Autodesk Inventor part; units mm, degrees
ref_plane "YZ Plane" through (0, 0, 0) normal (1, 0, 0) x (0, 1, 0)
ref_plane "XZ Plane" through (0, 0, 0) normal (0, 1, 0) x (-1, 0, 0)
ref_plane "XY Plane" through (0, 0, 0) normal (0, 0, 1) x (1, 0, 0)
sketch "Sketch1" plane through (0, 0, 0) normal (0, 0, 1) x (1, 0, 0)
  line L0 (0, 0) -> (20, 0)
  line L1 (20, 0) -> (20, -16)
  line L2 (20, -16) -> (0, -16)
  line L3 (0, -16) -> (0, 0)
  circle A0 centre (10, -8) radius 2.5
  dimension "d0" = 20
  dimension "d1" = 16
  dimension "d2" = 8
  dimension "d3" = 10
  dimension "d4" = 5
extrude "Extrusion1" add sketch "Sketch1" along normal blind 5
sketch "Sketch2" plane through (0, 0, 0) normal (0, 1, 0) x (1, 0, 0)
  line L0 (20, 0) -> (20, -5)
  line L1 (20, 0) -> (30, 0)
  line L2 (30, 0) -> (30, 7.76)
  line L3 (30, 7.76) -> (20, 7.76)
  line L4 (20, 7.76) -> (20, 0)
  line L5 (20, -5) -> (30, -5)
  line L6 (30, -5) -> (30, 0)
  line L7 (30, 0) -> (20, 0)
  line L8 (20, 0) -> (20, -5)
  circle A0 centre (25, 3.88) radius 2.6
  point P0 (0, 0)
  dimension "d7" = 10
  dimension "d8" = 7.76
  dimension "d9" = 5.2
extrude "Extrusion2" add sketch "Sketch2" against normal blind 16
sketch "Sketch3" plane through (0, -16, 0) normal (0, -1, 0) x (1, 0, 0)
  line L0 (30, -7.76) -> (30, 5)
  line L1 (0, 0) -> (20, 0)
  line L2 (30, -7.76) -> (20, -7.76)
  line L3 (20, -7.76) -> (20, 0)
  line L4 (20, 0) -> (30, 0)
  line L5 (30, 0) -> (30, -7.76)
extrude "Extrusion3" add sketch "Sketch3" against normal blind 9
sketch "Sketch4" plane through (0, -16, 0) normal (0, -1, 0) x (1, 0, 0)
  circle A0 centre (25, -3.88) radius 2.6
  circle A1 centre (25, -3.88) radius 2.6
  point P0 (0, 0)
  dimension "d16" = 5.2
extrude "Extrusion4" cut sketch "Sketch4" against normal blind 5
properties part number "cover mount LR v02"
Verification items for the finished model (mm, model axes). A direction names the side the tool comes from. Coordinates: 2 decimals unless noted, no trailing zeros. Order: outer loops, then holes, each group sorted by start corner. A loop starts at its lowest first (then second) coordinate and runs counter-clockwise, first axis right, second up. Notation, with made-up numbers: (-24.5, 25) -> (-16.5, 25) arc R20 ccw to (-16.5, 31) -> close; hole circle Ø4 at (5, -18.5). An arc over 180 degrees is marked (long way). Answer as CSV lines item,"result". Start each with the question number.
1) Cross-section at B-B, the plane x = 10. Record the boundary of the cut face in (y, z), then the cut area to 3 significant figures.
2) Material ranges on L1, parallel to Z at x = 25, y = -1.75; L2, parallel to X at y = -2.25, z = -3.88; L3, parallel to Y at x = 24, z = -4.5, recorded low to high. Write a range as [from, to].
3) Release check for a two-part mould opening along Z. For faces 4 (the face through (12, -6, 0)), 5 (the face through (15, -8, 5)), 6 (the face through (24.44, -13.54, -6.42)), 7 (the face through (24.44, -3.45, -1.34)) record: released by +Z, released by -Z, zero draft, split by the parting line, or undercut.
4) Set-up check for faces 1 (the face through (25, -11, -4)), 2 (the face through (25, -7, -4)), 3 (the face through (20, -8, -4)): record each of +Z, -Z, +X, -X, +Y, -Y from which the full face is reachable in a straight line by a thin tool's end or side.
5) Cross-section at A-A, the plane y = -8. Record the boundary of the cut face in (x, z).
6) Cross-section at D-D, the plane z = 1.75. Record the boundary of the cut face in (x, y).
7) Cross-section at C-C, the plane y = -11.75. Record the boundary of the cut face in (x, z).
8) Gauge pin test, flat ends, axial feed: pin 1 Ø3 at (x, y) = (3.5, -7.5) entering from -Z; pin 2 Ø3 at (x, z) = (25, -3.88) entering from +Y; pin 3 Ø2.5 at (x, z) = (26, -4) entering from -Y. Record the tip position at first contact, or that the pin passes through.
Conclusion:
1,outline,"(-16, 0) -> (-10.5, 0) -> (-10.5, 5) -> (-16, 5) -> close; (-5.5, 0) -> (0, 0) -> (0, 5) -> (-5.5, 5) -> close"
1,area,"55.0 mm²"
2,L1,"z = [-7.76, -6.48], [-1.28, 5]"
2,L2,"x = [20, 22.4], [27.6, 30]"
2,L3,"y = [-11, -7]"
3,face 4,"released by -Z"
3,face 5,"released by +Z"
3,face 6,"undercut"
3,face 7,"undercut"
4,face 1,"-Y"
4,face 2,"+Y"
4,face 3,"-Z, -X, +Y, -Y"
5,outline,"(0, 0) -> (7.5, 0) -> (7.5, 5) -> (0, 5) -> close; (12.5, 0) -> (20, 0) -> (20, -7.76) -> (30, -7.76) -> (30, 5) -> (12.5, 5) -> close"
6,outline,"(0, -16) -> (30, -16) -> (30, 0) -> (0, 0) -> close; hole circle Ø5 at (10, -8)"
7,outline,"(0, 0) -> (20, 0) -> (20, -7.76) -> (30, -7.76) -> (30, 5) -> (0, 5) -> close; hole circle Ø5.2 at (25, -3.88)"
8,pin 1,"stops at z = 0"
8,pin 2,"stops at y = -7"
8,pin 3,"stops at y = -11"
